Could you check a few things on this model? Use its own coordinates, in mm. Round coordinates to 2 decimals unless told otherwise and drop trailing zeros. Loops run counter-clockwise (first coordinate to the right, second up) from the corner with the lowest first, then second, coordinate; pieces in that order, holes last. Notation, with made-up numbers: (70.25, -13) -> (112.25, -13) arc R27 ccw to (112.25, 10) -> close; hole circle Ø3 at (-6, -26.75). An arc over 180 degrees is marked (long way). Use CSV: the item, a comma, the result in double quotes. Start each with the question number.
```python
from build123d import *

# Parameters (mm, degrees)
BOSS_EXTRU_2_DEPTH      = 5.1
BOSS_EXTRU_2_DEPTH_BACK = 5.1
ESQUISSE9_R             = 12
ESQUISSE10_R            = 2.5
ENL_V_MAT_EXTRU_3_DEPTH = 20.8
CONG_1_R                = 0.15
ESQUISSE13_R            = 8
ESQUISSE13_R_2          = 6
ENL_V_MAT_EXTRU_4_DEPTH = 0.01
ENL_V_START             = -0.01
ESQUISSE14_R            = 8
ESQUISSE14_R_2          = 6
ENL_V_MAT_EXTRU_5_DEPTH = 0.01


with BuildPart() as part:
    # Esquisse9 → Boss.-Extru.2 (new, two sides: drawn at the far end of the back side and taken through both)
    with BuildSketch(Plane(origin=(5.1, 0, 0), x_dir=(0, 0, -1), z_dir=(1, 0, 0)).offset(-BOSS_EXTRU_2_DEPTH_BACK)):
        Circle(ESQUISSE9_R)
    extrude(amount=BOSS_EXTRU_2_DEPTH + BOSS_EXTRU_2_DEPTH_BACK)

    # Esquisse10 → Enl_v. mat.-Extru.3 (cut, through all)
    with BuildSketch(Plane(origin=(10.2, 0, 0), x_dir=(0, 0, -1), z_dir=(1, 0, 0))):
        Circle(ESQUISSE10_R)
    extrude(amount=-ENL_V_MAT_EXTRU_3_DEPTH, mode=Mode.SUBTRACT)

    # Esquisse11 → Enl_vement de mati_re-R_volution1 (revolve, cut)
    with BuildSketch(Plane.XY, mode=Mode.PRIVATE) as enl_vement_de_mati_re_r_volution1_sk:
        Polygon((0, -9.003888398), (2.102617573, -12), (8.097659703, -12), (10.2, -9.003888398), (10.2, -12), (7.948691549, -12.31078505), (2.020448567, -12.31078505), (0, -12), align=None)
        Polygon((10.2, 12), (7.948691549, 12.31078505), (2.020448567, 12.31078505), (0, 12), (0, 9.003888398), (2.102617573, 12), (8.097659703, 12), (10.2, 9.003888398), align=None)
    revolve(enl_vement_de_mati_re_r_volution1_sk.sketch.rotate(Axis((10.2, 0, 0), (-1, 0, 0)), 180), axis=Axis((10.2, 0, 0), (-1, 0, 0)), mode=Mode.SUBTRACT)

    # Cong_1
    cong_1_edges = [part.edges().sort_by_distance(p)[0] for p in [
        (10.2, 0, 2.5),
    ]]
    fillet(cong_1_edges, radius=CONG_1_R)

    # Esquisse13 → Enl_v. mat.-Extru.4 (cut)
    with BuildSketch(Plane(origin=(10.2, 0, 0), x_dir=(0, 0, -1), z_dir=(1, 0, 0))):
        Circle(ESQUISSE13_R)
        Circle(ESQUISSE13_R_2, mode=Mode.SUBTRACT)
    extrude(amount=-ENL_V_MAT_EXTRU_4_DEPTH, mode=Mode.SUBTRACT)

    # Esquisse14 → Enl_v. mat.-Extru.5 (cut)
    with BuildSketch(Plane.ZY.offset(ENL_V_START)):
        with Locations(Location((0, 0, 0), (0, 0, 180))):
            Circle(ESQUISSE14_R)
        with Locations(Location((0, 0, 0), (0, 0, 180))):
            Circle(ESQUISSE14_R_2, mode=Mode.SUBTRACT)
    extrude(amount=ENL_V_MAT_EXTRU_5_DEPTH, mode=Mode.SUBTRACT)


solid = part.part
```
1. Will these pins go through, and if not, where does the flat tip stop? pin 1 (4 mm diameter, centred on x = 2.5, z = -6.5, fed in from -Y); pin 2 (5 mm diameter, centred on x = 5.5, y = 3, fed in from +Z); pin 3 (4 mm diameter, centred on x = 3, z = -8, fed in from +Y).
2. Suppose I cut it at C-C (x = 4.75). List the corners of the cut face in (y, z) for me.
3. If I drill on L1, parallel to X at y = -6.5, z = -2.25; L2, parallel to Y at x = 2.5, z = 2; L3, parallel to Z at x = 6, y = 6.75, over which ranges is the centre line in solid material (lowest first)?
4. Suppose I cut it at D-D (x = 8.5). List the corners of the cut face in (y, z) for me, then the cut area to 3 significant figures.
Geometry check:
1,pin 1,"stops at y = -11.12"
1,pin 2,"stops at z = 11.99"
1,pin 3,"stops at y = 10.39"
2,outline,"circle Ø24 at (0, 0); hole circle Ø5 at (0, 0)"
3,L1,"x = 0.01 to 10.19"
3,L2,"y = -11.83 to -1.5, 1.5 to 11.83"
3,L3,"z = -9.92 to 9.92"
4,outline,"circle Ø22.85 at (0, 0); hole circle Ø5 at (0, 0)"
4,area,"391 mm²"
